Design review of the part built by this model. Coordinates are the model's own, in mm. Face numbers are marked on the shaded views. A direction names the side the tool comes from. Give positions to 0.01 mm unless a question says otherwise; leave off trailing zeros. Write each loop counter-clockwise with the first axis right and the second up, starting at its lowest first coordinate (ties: lowest second). Pieces come first, ordered by that corner, then holes. Notation, with made-up numbers: M -8,82 L 5,82 A20 cw 5,108 Z; hole C 73.25,5 d6. An arc over 180 degrees is marked long. Use a Markdown table: item, result. Add a question column.
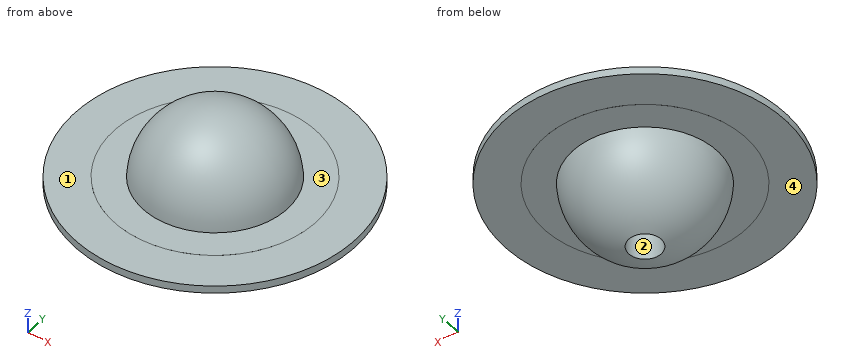
Solid Edge part; units mm, degrees
sketch "Sketch1" plane through (0, 0, 0) normal (0, -1, 0) x (1, 0, 0)
  line L0 (0, 22.6935) -> (0, -22.6935)
  arc A0 (0, 22.6935) -> (0, -22.6935) centre (0, 0) cw
revolve "RevolvedProtrusion1" add sketch "Sketch1" angle 360 about axis through (0, 0, 22.6935) along (0, 0, -1)
sketch "Sketch2" plane through (0, 0, 0) normal (0, 0, 1) x (1, 0, 0)
  circle A0 centre (0, 0) radius 44
extrude "Protrusion1" add sketch "Sketch2" along normal mid plane 2.35
sketch "Sketch3" plane through (0, 0, 0) normal (0, 0, 1) x (1, 0, 0)
  circle A0 centre (0, 0) radius 31.7083
extrude "ExtrudedProtrusion_9" add sketch "Sketch3" along normal mid plane 2.36
sketch "Sketch4" plane through (0, 0, 0) normal (0, 0, 1) x (1, 0, 0)
  circle A0 centre (0, 0) radius 5.09
extrude "ExtrudedCutout_1" cut sketch "Sketch4" against normal blind 53.2556
(1) Machinability: for the marked faces 3 and 4, which of the approach directions +Z, -Z, +X, -X, +Y, -Y give a long, thin tool a straight path to every point of the face, cutting with its end or side? Answer none if there is none.
(2) Add section C-C on z = 12. Give the boundary of the cut face in (x, y).
(3) The part is to be moulded in two halves that separate along X. For the marked faces 1 and 2, say which applies: released by +X, released by -X, zero draft, split by the parting line, or undercut.
(4) For pin 1 (8 mm diameter, centred on x = -0.5, y = 1.5, fed in from -Z); pin 2 (8 mm diameter, centred on x = -23, y = 2.5, fed in from -Z); pin 3 (1 mm diameter, centred on x = 13.5, z = 5.5, fed in from -Y); pin 4 (10 mm diameter, centred on y = 26, z = 10, fed in from +X), all flat-tipped, find the tip position at first contact; note any pin that passes through.
(5) Wall thickness on L1, parallel to Z at x = -31.5, y = -28.5 (3 decimals); L2, parallel to Y at x = 0, z = -11; L3, parallel to X at y = -4, z = -11.5: over which ranges is each line inside the solid? List them lowest first.
(6) Add section D-D on x = -30.5. Give the boundary of the cut face in (y, z) (3 decimals).
From the geometry:
| question | item | result |
|---|---|---|
| 1 | face 3 | +Z |
| 1 | face 4 | -Z |
| 2 | outline | C 0,0 d38.52 |
| 3 | face 1 | zero draft |
| 3 | face 2 | undercut |
| 4 | pin 1 | stops at z = -22.12 |
| 4 | pin 2 | stops at z = -12.2 |
| 4 | pin 3 | stops at y = -17.8 |
| 4 | pin 4 | passes through |
| 5 | L1 | z = -1.175 to 1.175 |
| 5 | L2 | y = -19.85 to -5.09, 5.09 to 19.85 |
| 5 | L3 | x = -19.15 to -3.15, 3.15 to 19.15 |
| 6 | outline | M -31.714,-1.175 L -8.67,-1.175 L -8.67,-1.18 L 8.67,-1.18 L 8.67,-1.175 L 31.714,-1.175 L 31.714,1.175 L 8.67,1.175 L 8.67,1.18 L -8.67,1.18 L -8.67,1.175 L -31.714,1.175 Z |
